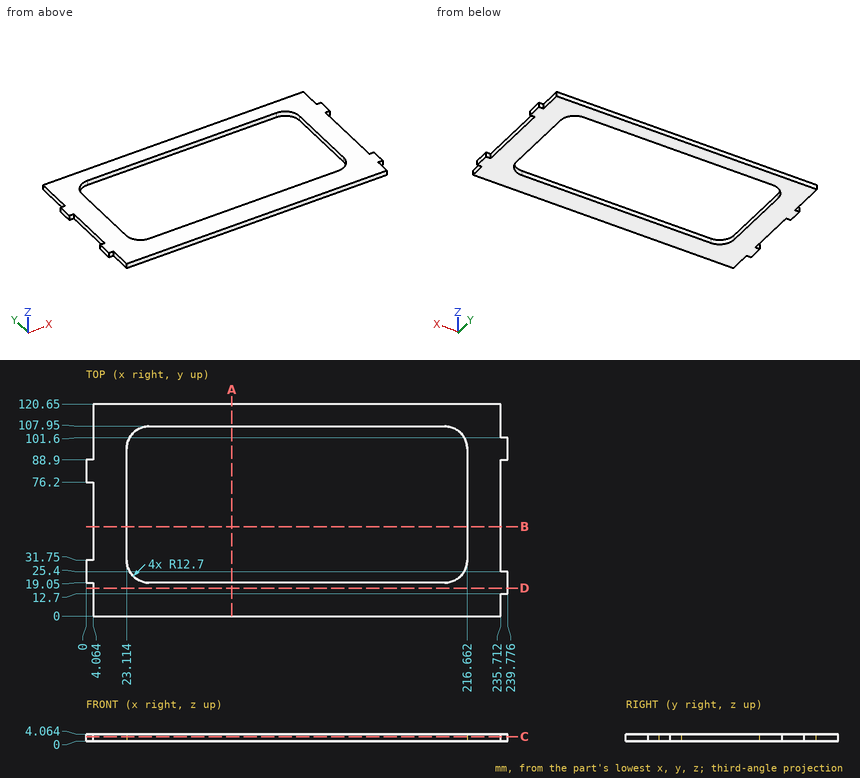
Job drawing, mm, ordinate dimensions from the low corner. One solid piece. Give positions to 0.01 mm unless a question says otherwise; leave off trailing zeros. Write each loop counter-clockwise with the first axis right and the second up, starting at its lowest first coordinate (ties: lowest second). Pieces come first, ordered by that corner, then holes. Notation, with made-up numbers: (73, -9.75) - (99, -9.75) arc R29 cw to (99, 24.25) - close; hole circle Ø1 at (37.25, -26.75). An arc over 180 degrees is marked (long way). Use one line per item in the form item = value. Start each with the question number.
1. Band-saw the part on A-A on x = 83. Write the cut outline in (y, z), plus the area to 3 significant figures.
2. Band-saw the part on B-B on y = 51. Write the cut outline in (x, z).
3. Band-saw the part on C-C on z = 2.65. Write the cut outline in (x, y).
4. Drop flat-ended pins along their axis: pin 1 Ø2 at (y, z) = (112.5, 2) entering from -X; pin 2 Ø1.2 at (x, z) = (2, 2) entering from +Y; pin 3 Ø3 at (x, y) = (130.5, 14) entering from -Z; pin 4 Ø1.2 at (y, z) = (47, 1) entering from +X. Give the stop position or say it passes through.
5. Band-saw the part on D-D on y = 16. Write the cut outline in (x, z), plus the area to 3 significant figures.
6. Probe line 1 (X direction, y = 47.5, z = 2.8); line 2 (Y direction, x = 126, z = 2.8); line 3 (X direction, y = 116, z = 0.2). List the from-to ranges inside material, lowest first. Write a range as [from, to].
Conclusion:
q1.outline = (0, 0) - (19.05, 0) - (19.05, 4.06) - (0, 4.06) - close; (107.95, 0) - (120.65, 0) - (120.65, 4.06) - (107.95, 4.06) - close
q1.area = 129 mm²
q2.outline = (4.06, 0) - (23.11, 0) - (23.11, 4.06) - (4.06, 4.06) - close; (216.66, 0) - (235.71, 0) - (235.71, 4.06) - (216.66, 4.06) - close
q3.outline = (0, 19.05) - (4.06, 19.05) - (4.06, 0) - (235.71, 0) - (235.71, 12.7) - (239.78, 12.7) - (239.78, 25.4) - (235.71, 25.4) - (235.71, 88.9) - (239.78, 88.9) - (239.78, 101.6) - (235.71, 101.6) - (235.71, 120.65) - (4.06, 120.65) - (4.06, 88.9) - (0, 88.9) - (0, 76.2) - (4.06, 76.2) - (4.06, 31.75) - (0, 31.75) - close; hole (23.11, 31.75) arc R12.7 ccw to (35.81, 19.05) - (203.96, 19.05) arc R12.7 ccw to (216.66, 31.75) - (216.66, 95.25) arc R12.7 ccw to (203.96, 107.95) - (35.81, 107.95) arc R12.7 ccw to (23.11, 95.25) - close
q4.pin_1 = 4.06
q4.pin_2 = 88.9
q4.pin_3 = 0
q4.pin_4 = 235.71
q5.outline = (4.06, 0) - (239.78, 0) - (239.78, 4.06) - (4.06, 4.06) - close
q5.area = 958 mm²
q6.line_1 = [4.06, 23.11], [216.66, 235.71]
q6.line_2 = [0, 19.05], [107.95, 120.65]
q6.line_3 = [4.06, 235.71]
